```python
from build123d import *

# Parameters (mm, degrees)
BOSS_EXTRUDE1_DEPTH                                = 25.4
FILLET1_R                                          = 127
FILLET2_R                                          = 25.4
WHEEL_SLOT_DEPTH                                   = 25.4
PEDAL_SLOT_DEPTH                                   = 25.4
BOSS_EXTRUDE2_DEPTH                                = 25.4
FILLET3_R                                          = 25.4
CSK_FOR_10_FLAT_HEAD_MACHINE_SCREW_100_D           = 5.1054
CSK_FOR_10_FLAT_HEAD_MACHINE_SCREW_100_CSINK_D     = 9.779
CSK_FOR_10_FLAT_HEAD_MACHINE_SCREW_100_CSINK_ANGLE = 100


# Read off the part's stored shape, not the designer's step: wheel slot, pedal slot
with BuildPart() as part:
    # Sketch1 → Boss-Extrude1 (new body)
    with BuildSketch(Plane.XY):
        Polygon((0, 0), (-193.132194655, 334.514773719), (-19.646968374, 635), (107.353031626, 635), (-11.089113546, 889), (-576.905448196, 889), (-897.037642851, 334.514773719), (-703.905448196, 0), align=None)
    extrude(amount=BOSS_EXTRUDE1_DEPTH)

    # Fillet1
    fillet1_edges = [part.edges().sort_by_distance(p)[0] for p in [
        (-897.037642851, 334.514773719, 12.7),
        (-193.132194655, 334.514773719, 12.7),
    ]]
    fillet(fillet1_edges, radius=FILLET1_R)

    # Fillet2
    fillet2_edges = [part.edges().sort_by_distance(p)[0] for p in [
        (-576.905448196, 889, 12.7),
        (-11.089113546, 889, 12.7),
        (107.353031626, 635, 12.7),
        (-19.646968374, 635, 12.7),
    ]]
    fillet(fillet2_edges, radius=FILLET2_R)

    # wheel slot outline → wheel slot (cut)
    with BuildSketch(Plane.XY):
        with BuildLine():
            Line((-154.207271537, 714.375), (-154.207271537, 809.625))
            ThreePointArc((-154.207271537, 809.625), (-157.382271537, 812.8), (-160.557271537, 809.625))
            Line((-160.557271537, 809.625), (-160.557271537, 714.375))
            ThreePointArc((-160.557271537, 714.375), (-157.382271537, 711.2), (-154.207271537, 714.375))
        make_face()
        with BuildLine():
            Line((-27.207271537, 714.375), (-27.207271537, 809.625))
            ThreePointArc((-27.207271537, 809.625), (-30.382271537, 812.8), (-33.557271537, 809.625))
            Line((-33.557271537, 809.625), (-33.557271537, 714.375))
            ThreePointArc((-33.557271537, 714.375), (-30.382271537, 711.2), (-27.207271537, 714.375))
        make_face()
    extrude(amount=WHEEL_SLOT_DEPTH, mode=Mode.SUBTRACT)

    # pedal slot outline → pedal slot (cut)
    with BuildSketch(Plane.XY):
        with BuildLine():
            Line((-720.725, 352.425), (-295.275, 352.425))
            ThreePointArc((-295.275, 352.425), (-292.1, 355.6), (-295.275, 358.775))
            Line((-295.275, 358.775), (-720.725, 358.775))
            ThreePointArc((-720.725, 358.775), (-723.9, 355.6), (-720.725, 352.425))
        make_face()
        with BuildLine():
            Line((-688.030448196, 260.789543073), (-262.580448196, 260.789543073))
            ThreePointArc((-262.580448196, 260.789543073), (-259.405448196, 263.964543073), (-262.580448196, 267.139543073))
            Line((-262.580448196, 267.139543073), (-688.030448196, 267.139543073))
            ThreePointArc((-688.030448196, 267.139543073), (-691.205448196, 263.964543073), (-688.030448196, 260.789543073))
        make_face()
        with BuildLine():
            Line((-637.230448196, 172.801362049), (-211.780448196, 172.801362049))
            ThreePointArc((-211.780448196, 172.801362049), (-208.605448196, 175.976362049), (-211.780448196, 179.151362049))
            Line((-211.780448196, 179.151362049), (-637.230448196, 179.151362049))
            ThreePointArc((-637.230448196, 179.151362049), (-640.405448196, 175.976362049), (-637.230448196, 172.801362049))
        make_face()
    extrude(amount=PEDAL_SLOT_DEPTH, mode=Mode.SUBTRACT)

    # Sketch6 → Boss-Extrude2 (add)
    with BuildSketch(Plane.XY.offset(25.4)):
        with BuildLine():
            Line((0, 0), (812.8, 0))
            Line((812.8, 0), (812.8, 508))
            Line((812.8, 508), (-16.622799945, 508))
            Line((-16.622799945, 508), (-54.796626253, 574.119006685))
            Line((-54.796626253, 574.119006685), (-156.470452561, 398.014773719))
            ThreePointArc((-156.470452561, 398.014773719), (-173.485226281, 334.514773719), (-156.470452561, 271.014773719))
            Line((-156.470452561, 271.014773719), (0, 0))
        make_face()
    extrude(amount=-BOSS_EXTRUDE2_DEPTH)

    # Fillet3
    fillet3_edges = [part.edges().sort_by_distance(p)[0] for p in [
        (-54.796626253, 574.119006685, 12.7),
        (-16.622799945, 508, 12.7),
    ]]
    fillet(fillet3_edges, radius=FILLET3_R)

    # CSK for #10 Flat Head Machine Screw (100)1 (through all)
    with Locations(Plane.XY.offset(25.4)):
        with Locations((-524.140751359, 876.3), (-524.140751359, 825.5), (-492.390751359, 876.3), (-441.590751359, 876.3), (-390.790751359, 876.3), (-339.990751359, 876.3), (-289.190751359, 876.3), (-238.390751359, 876.3), (-524.140751359, 774.7), (-524.140751359, 723.9), (-524.140751359, 673.1), (-524.140751359, 622.3), (-524.140751359, 571.5), (-187.590751359, 876.3)):
            CounterSinkHole(CSK_FOR_10_FLAT_HEAD_MACHINE_SCREW_100_D / 2, CSK_FOR_10_FLAT_HEAD_MACHINE_SCREW_100_CSINK_D / 2, counter_sink_angle=CSK_FOR_10_FLAT_HEAD_MACHINE_SCREW_100_CSINK_ANGLE)


solid = part.part
```
Work out the finished part from the listing and answer in its coordinate system (mm). Round coordinates to 2 decimals unless told otherwise and drop trailing zeros. Loops run counter-clockwise (first coordinate to the right, second up) from the corner with the lowest first, then second, coordinate; pieces in that order, holes last. Notation, with made-up numbers: (30.25, -17.5) -> (66.25, -17.5) arc R20 ccw to (66.25, -4.5) -> close; hole circle Ø4 at (36, -38). An arc over 180 degrees is marked (long way). Write each question's results on one line, items separated by ' | '. Start each with the question number.
1. Section B-B (z = 11.75) is taken. State how many separate pieces and enclosed holes the cut face has, plus the area to 3 significant figures.
2. Given pin 1 Ø6 at (x, y) = (-524.14, 622.3) entering from +Z; pin 2 Ø3 at (x, y) = (-289.19, 876.3) entering from -Z; pin 3 Ø5 at (y, z) = (752, 22) entering from +X; pin 4 Ø1 at (x, z) = (533.5, 20) entering from +Y, each flat-ended and moving along its own axis, determine where each tip first touches the part or whether it passes through.
3. Find the intervals of material crossed by probe 1 along Y at (x, z) = (-279, 7.25); probe 2 along Y at (x, z) = (361, 2.5); probe 3 along X at (y, z) = (825.5, 13.25), in increasing order. Write a range as from..to.
4. Section C-C (y = 461.5) is taken. Determine the outline of the cut face in (x, z), plus the area to 3 significant figures.
5. Section A-A (x = 222) is taken. Determine the outline of the cut face in (y, z), plus the area to 3 significant figures.
Evaluation:
1) separate pieces: 1 | enclosed holes: 19 | area: 1,090,000 mm2
2) pin 1: stops at z = 23.82 | pin 2: passes through | pin 3: stops at x = 53.96 | pin 4: stops at y = 508
3) probe 1: y = 0..172.8, 179.15..260.79, 267.14..889 | probe 2: y = 0..508 | probe 3: x = -613.57..-526.69, -521.59..18.52
4) outline: (-823.72, 0) -> (812.8, 0) -> (812.8, 25.4) -> (-823.72, 25.4) -> close | area: 41,600 mm2
5) outline: (0, 0) -> (508, 0) -> (508, 25.4) -> (0, 25.4) -> close | area: 12,900 mm2
